from build123d import *

# Parameters (mm, degrees)
SKETCH1_W           = 78
SKETCH1_H           = 48
BOSS_EXTRUDE1_DEPTH = 30
CHAMFER1_SIZE       = 5
CUT_EXTRUDE1_DEPTH  = 87.948260477
CUT_EXTRUDE2_DEPTH  = 101.553903722


with BuildPart() as part:
    # Sketch1 → Boss-Extrude1 (new body)
    with BuildSketch(Plane(origin=(0, 0, 0), x_dir=(1, 0, 0), z_dir=(0, 1, 0))):
        with Locations((39, 0)):
            Rectangle(SKETCH1_W, SKETCH1_H)
    extrude(amount=BOSS_EXTRUDE1_DEPTH)

    # Chamfer1
    chamfer1_edges = [part.edges().sort_by_distance(p)[0] for p in [
        (0, 30, 0),
    ]]
    chamfer(chamfer1_edges, length=CHAMFER1_SIZE)

    # Sketch2 → Cut-Extrude1 (cut, through all)
    with BuildSketch(Plane(origin=(0, 30, 0), x_dir=(1, 0, 0), z_dir=(0, 1, 0))):
        with BuildLine():
            Line((18, 6), (36, 6))
            ThreePointArc((36, 6), (42, 0), (36, -6))
            Line((36, -6), (18, -6))
            ThreePointArc((18, -6), (12, 0), (18, 6))
        make_face()
    extrude(amount=-CUT_EXTRUDE1_DEPTH, mode=Mode.SUBTRACT)

    # Sketch3 → Cut-Extrude2 (cut, through all, along a direction that is not the sketch's normal)
    with BuildSketch(Plane(origin=(0, 30, 0), x_dir=(1, 0, 0), z_dir=(0, 1, 0))):
        Polygon((78, 24), (66.124355653, 24), (54, 3), (48, 3), (48, -3), (54, -3), (66.124355653, -24), (78, -24), align=None)
    extrude(amount=-CUT_EXTRUDE2_DEPTH, dir=(-0.5000000000000044, 0.8660254037844362, 0), mode=Mode.SUBTRACT)


solid = part.part
Design review of the part built by this model. Coordinates are the model's own, in mm. A direction names the side the tool comes from. Round coordinates to 2 decimals unless told otherwise and drop trailing zeros. Write each loop counter-clockwise with the first axis right and the second up, starting at its lowest first coordinate (ties: lowest second). Pieces come first, ordered by that corner, then holes. Notation, with made-up numbers: (-5, 39.25) -> (8, 39.25) arc R15 cw to (8, 62.25) -> close; hole circle Ø9 at (40.25, -7). An arc over 180 degrees is marked (long way). One line per question, with ' | ' between items.
(1) Draft analysis for pull direction Z (two halves, no side actions). For faces 1 (the flat face through (38, 15, -24)), 2 (the flat face through (42, 30, -6)), 3 (the flat face through (68.06, 15.21, -12.56)), 4 (the flat face through (38, 15, 24)), state which applies: released by +Z, released by -Z, zero draft, split by the parting line, or undercut.
Result sheet:
face 1: released by -Z | face 2: zero draft | face 3: undercut | face 4: released by +Z
(2) Wall thickness on line 1 (Z direction, x = 35, y = 22.5); line 2 (Z direction, x = 52, y = 27); line 3 (X direction, y = 11, z = -3.5): over which ranges is each line inside the solid? List them lowest first. Write a range as [from, to].
Result sheet:
line 1: [-24, -6], [6, 24] | line 2: [-24, -3], [3, 24] | line 3: [0, 13.13], [40.87, 65.26]
(3) Take a section at C-C, the plane y = 26.5. State the section outline as (x, z) points.
Result sheet:
outline: (1.5, -24) -> (68.15, -24) -> (56.02, -3) -> (50.02, -3) -> (50.02, 3) -> (56.02, 3) -> (68.15, 24) -> (1.5, 24) -> close; hole (18, -6) -> (36, -6) arc R6 ccw to (36, 6) -> (18, 6) arc R6 ccw to start
(4) Take a section at D-D, the plane z = 5. State the section outline as (x, y) points, and give its area (3 significant figures).
Result sheet:
outline: (0, 0) -> (14.68, 0) -> (14.68, 30) -> (5, 30) -> (0, 25) -> close; (39.32, 0) -> (72.48, 0) -> (55.15, 30) -> (39.32, 30) -> close | area: 1,160 mm2
(5) Insertion check: P1, Ø4, axis at y = 18.5, z = -14.5, coming from the +X side; P2, Ø8, axis at y = 24.5, z = -9.5, coming from the +X side; P3, Ø5, axis at x = 47, z = 4, coming from the -Y side. Each pin has a flat end and moves straight along its axis. Give the tip position at first contact, or say it passes through.
Result sheet:
P1: x = 68.91 | P2: x = 64.19 | P3: y = 0
(6) Machinability: for faces 5 (the flat face through (56.54, 15.21, -0.04)), 6 (the flat face through (78, 4, 20)), 7 (the cylindrical face through (42, 15, 0)), which of the approach directions +Z, -Z, +X, -X, +Y, -Y give a long, thin tool a straight path to every point of the face, cutting with its end or side? Answer none if there is none.
Result sheet:
face 5: +X, +Y | face 6: +Z, -Z, +X, +Y, -Y | face 7: +Y, -Y
(7) Take a section at B-B, the plane z = 0. State the section outline as (x, y) points, and give its area (3 significant figures).
Result sheet:
outline: (0, 0) -> (12, 0) -> (12, 30) -> (5, 30) -> (0, 25) -> close; (42, 0) -> (65.32, 0) -> (48, 30) -> (42, 30) -> close | area: 787 mm2
(8) Take a section at A-A, the plane x = 22. State the section outline as (y, z) points, and give its area (3 significant figures).
Result sheet:
outline: (0, -24) -> (30, -24) -> (30, -6) -> (0, -6) -> close; (0, 6) -> (30, 6) -> (30, 24) -> (0, 24) -> close | area: 1,080 mm2
